```python
from build123d import *

# Parameters (mm, degrees)
F0_W          = 350
F0_H          = 20
F1_DEPTH      = 10
F1_DEPTH_BACK = 10
F2_R          = 8.5
F3_DEPTH      = 355.6


with BuildPart() as f1:
    # F0 (on Top) → F1 (new body, two sides)
    with BuildSketch(Plane.XY) as f1_sk:
        Rectangle(F0_W, F0_H)
    extrude(amount=F1_DEPTH)
    extrude(f1_sk.sketch, amount=-F1_DEPTH_BACK)

    # F2 (on face) → F3 (cut)
    with BuildSketch(Plane(origin=(-175, 0, 0), x_dir=(0, -1, 0), z_dir=(-1, 0, 0))):
        with BuildLine():
            ThreePointArc((0, 10), (7.071068, 7.071068), (10, 0))
            Line((10, 0), (10, 10))
            Line((10, 10), (0, 10))
        make_face()
        with BuildLine():
            Line((10, -10), (10, 0))
            ThreePointArc((10, 0), (7.071068, -7.071068), (0, -10))
            Line((0, -10), (10, -10))
        make_face()
        with BuildLine():
            ThreePointArc((-10, 0), (-7.071068, 7.071068), (0, 10))
            Line((0, 10), (-10, 10))
            Line((-10, 10), (-10, 0))
        make_face()
        with BuildLine():
            Line((-10, -10), (0, -10))
            ThreePointArc((0, -10), (-7.071068, -7.071068), (-10, 0))
            Line((-10, 0), (-10, -10))
        make_face()
        Circle(F2_R)
    extrude(amount=-F3_DEPTH, mode=Mode.SUBTRACT)


solid = f1.part
```
Geometry: final body of the model. Coordinates: model frame, mm. Give positions to 0.01 mm unless a question says otherwise; leave off trailing zeros. Loops run counter-clockwise (first coordinate to the right, second up) from the corner with the lowest first, then second, coordinate; pieces in that order, holes last. Notation, with made-up numbers: (80, 4.25) - (136, 4.25) arc R27 ccw to (136, 35.25) - close; hole circle Ø11 at (27, 40.25). An arc over 180 degrees is marked (long way). Answer as CSV lines item,"result". Start each with the question number.
(1) Pin query (flat end, axial travel): P1, Ø4, axis at x = -103.5, z = -4, coming from the +Y side; P2, Ø1, axis at x = -14.5, y = 1, coming from the +Z side; P3, Ø5, axis at y = 4.5, z = -2.5, coming from the +X side; P4, Ø5, axis at x = -136.5, z = -6.5, coming from the -Y side. Return the tip coordinate at first contact, or that it passes through.
(2) Mould query, pull axis Z, two halves, no side actions, for faces 1 (the face through (-2.45, -4.57, 7.167)), 2 (the face through (-175, -4.5, -7.4)). Classes: +Z half, -Z half, draft (parallel to the pull), parting line (faces both ways), or undercut.
(3) Ray query, line 1 along Z through (x, y) = (-141, 0.75); line 2 along Z through (x, y) = (-121.5, -1); line 3 along Y through (x, z) = (148.5, 1.25). Return the intervals inside material, ascending. Write a range as [from, to].
(4) Section query A-A (z = 5.25). Output: boundary loops of the cut face in (x, y).
(5) Section query B-B (x = -24). Output: boundary loops of the cut face in (y, z).
Worked answers:
1,P1,"stops at y = 9.8"
1,P2,"stops at z = 9.99"
1,P3,"passes through"
1,P4,"stops at y = -9.17"
2,face 1,"undercut"
2,face 2,"draft"
3,line 1,"z = [-9.97, -8.47], [8.47, 9.97]"
3,line 2,"z = [-9.95, -8.44], [8.44, 9.95]"
3,line 3,"y = [-9.92, -8.41], [8.41, 9.92]"
4,outline,"(-175, -8.51) - (175, -8.51) - (175, -6.68) - (-175, -6.68) - close; (-175, 6.68) - (175, 6.68) - (175, 8.51) - (-175, 8.51) - close"
5,outline,"(-10, 0) arc R10 ccw to (0, -10) arc R10 ccw to (10, 0) arc R10 ccw to (0, 10) arc R10 ccw to start; hole circle Ø17 at (0, 0)"
